```python
from build123d import *

# Parameters (mm, degrees)
SKETCH2_W                     = 520
SKETCH2_H                     = 70
BASE_FLANGE1_DEPTH            = 1
EDGE_FLANGE4_STRIP_W          = 5.4732
EDGE_FLANGE4_STRIP_H          = 1
EDGE_FLANGE4_STRIP_CUT_DEPTH  = 520
EDGE_FLANGE4_DEPTH            = 520
EDGE_FLANGE5_STRIP_W          = 5.4732
EDGE_FLANGE5_STRIP_H          = 1
EDGE_FLANGE5_STRIP_CUT_DEPTH  = 520
EDGE_FLANGE5_DEPTH            = 520
EDGE_FLANGE6_STRIP_W          = 5.4732
EDGE_FLANGE6_STRIP_H          = 1
EDGE_FLANGE6_STRIP_CUT_DEPTH  = 520
EDGE_FLANGE6_DEPTH            = 520
EDGE_FLANGE7_STRIP_W          = 5.4732
EDGE_FLANGE7_STRIP_H          = 1
EDGE_FLANGE7_STRIP_CUT_DEPTH  = 520
EDGE_FLANGE7_DEPTH            = 520
EDGE_FLANGE8_STRIP_W          = 5.4732
EDGE_FLANGE8_STRIP_H          = 1
EDGE_FLANGE8_STRIP_CUT_DEPTH  = 520
EDGE_FLANGE8_DEPTH            = 520
EDGE_FLANGE9_STRIP_W          = 5.4732
EDGE_FLANGE9_STRIP_H          = 1
EDGE_FLANGE9_STRIP_CUT_DEPTH  = 520
EDGE_FLANGE9_DEPTH            = 520
CUT_EXTRUDE2_REACH            = 527.071
CUT_EXTRUDE3_REACH            = 527.071
SKETCH38_R                    = 1.6
EDGE_FLANGE10_STRIP_W         = 5.4732
EDGE_FLANGE10_STRIP_H         = 1
EDGE_FLANGE10_STRIP_CUT_DEPTH = 520
EDGE_FLANGE10_DEPTH           = 520
HOLE1_START                   = 47
HOLE1_OUTLINE_R               = 1.5
HOLE1_DEPTH                   = 1
HOLE2_START                   = 47
HOLE2_OUTLINE_R               = 1.5
HOLE2_DEPTH                   = 1
HOLE3_START                   = -70
HOLE3_OUTLINE_R               = 1.5
HOLE3_DEPTH                   = 1
HOLE4_START                   = -70
HOLE4_OUTLINE_R               = 1.5
HOLE4_DEPTH                   = 1
SKETCH47_R                    = 1.5
CUT_EXTRUDE4_DEPTH            = 3


# Read off the part's stored shape, not the designer's step: Hole1, Hole2, Hole3, Hole4
# Sheet-metal steps are written as plain solids
with BuildPart() as part:
    # Sketch2 → Base-Flange1 (new body)
    with BuildSketch(Plane(origin=(0, 0, 0), x_dir=(1, 0, 0), z_dir=(0, 1, 0))):
        with Locations((260, 35)):
            Rectangle(SKETCH2_W, SKETCH2_H)
    extrude(amount=-BASE_FLANGE1_DEPTH)

    # Edge-Flange4 strip (across the edge) → Edge-Flange4 strip cut (cut)
    with BuildSketch(Plane(origin=(0, 0, 0), x_dir=(0, 0, -1), z_dir=(1, 0, 0))):
        with Locations((-1, -0.5)):
            Rectangle(EDGE_FLANGE4_STRIP_W, EDGE_FLANGE4_STRIP_H)
    extrude(amount=EDGE_FLANGE4_STRIP_CUT_DEPTH, mode=Mode.SUBTRACT)

    # Edge-Flange4 section (across the edge) → Edge-Flange4 (add)
    with BuildSketch(Plane(origin=(0, 0, 0), x_dir=(0, 0, -1), z_dir=(1, 0, 0))):
        with BuildLine():
            Line((0, 0.7366), (0, 14))
            Line((0, 14), (1, 14))
            Line((1, 14), (1, 0.7366))
            ThreePointArc((1, 0.7366), (1.215745145, 0.215745145), (1.7366, 0))
            Line((1.7366, 0), (1.7366, -1))
            ThreePointArc((1.7366, -1), (0.508638364, -0.491361636), (0, 0.7366))
        make_face()
    extrude(amount=EDGE_FLANGE4_DEPTH)

    # Edge-Flange5 strip (across the edge) → Edge-Flange5 strip cut (cut)
    with BuildSketch(Plane(origin=(520, 14, 0), x_dir=(0, -1, 0), z_dir=(-1, 0, 0))):
        with Locations((-1, -0.5)):
            Rectangle(EDGE_FLANGE5_STRIP_W, EDGE_FLANGE5_STRIP_H)
    extrude(amount=EDGE_FLANGE5_STRIP_CUT_DEPTH, mode=Mode.SUBTRACT)

    # Edge-Flange5 section (across the edge) → Edge-Flange5 (add)
    with BuildSketch(Plane(origin=(520, 14, 0), x_dir=(0, -1, 0), z_dir=(-1, 0, 0))):
        with BuildLine():
            Line((0, 0.7366), (0, 29))
            Line((0, 29), (1, 29))
            Line((1, 29), (1, 0.7366))
            ThreePointArc((1, 0.7366), (1.215745145, 0.215745145), (1.7366, 0))
            Line((1.7366, 0), (1.7366, -1))
            ThreePointArc((1.7366, -1), (0.508638364, -0.491361636), (0, 0.7366))
        make_face()
    extrude(amount=EDGE_FLANGE5_DEPTH)

    # Edge-Flange6 strip (across the edge) → Edge-Flange6 strip cut (cut)
    with BuildSketch(Plane(origin=(520, 13, 29), x_dir=(0, 0, -1), z_dir=(-1, 0, 0))):
        with Locations((-1, -0.5)):
            Rectangle(EDGE_FLANGE6_STRIP_W, EDGE_FLANGE6_STRIP_H)
    extrude(amount=EDGE_FLANGE6_STRIP_CUT_DEPTH, mode=Mode.SUBTRACT)

    # Edge-Flange6 section (across the edge) → Edge-Flange6 (add)
    with BuildSketch(Plane(origin=(520, 13, 29), x_dir=(0, 0, -1), z_dir=(-1, 0, 0))):
        with BuildLine():
            Line((0, 0.7366), (0, 14))
            Line((0, 14), (1, 14))
            Line((1, 14), (1, 0.7366))
            ThreePointArc((1, 0.7366), (1.215745145, 0.215745145), (1.7366, 0))
            Line((1.7366, 0), (1.7366, -1))
            ThreePointArc((1.7366, -1), (0.508638364, -0.491361636), (0, 0.7366))
        make_face()
    extrude(amount=EDGE_FLANGE6_DEPTH)

    # Edge-Flange7 strip (across the edge) → Edge-Flange7 strip cut (cut)
    with BuildSketch(Plane(origin=(0, -1, 29), x_dir=(0, 1, 0), z_dir=(1, 0, 0))):
        with Locations((-1, -0.5)):
            Rectangle(EDGE_FLANGE7_STRIP_W, EDGE_FLANGE7_STRIP_H)
    extrude(amount=EDGE_FLANGE7_STRIP_CUT_DEPTH, mode=Mode.SUBTRACT)

    # Edge-Flange7 section (across the edge) → Edge-Flange7 (add)
    with BuildSketch(Plane(origin=(0, -1, 29), x_dir=(0, 1, 0), z_dir=(1, 0, 0))):
        with BuildLine():
            Line((0, 0.7366), (0, 19))
            Line((0, 19), (1, 19))
            Line((1, 19), (1, 0.7366))
            ThreePointArc((1, 0.7366), (1.215745145, 0.215745145), (1.7366, 0))
            Line((1.7366, 0), (1.7366, -1))
            ThreePointArc((1.7366, -1), (0.508638364, -0.491361636), (0, 0.7366))
        make_face()
    extrude(amount=EDGE_FLANGE7_DEPTH)

    # Edge-Flange8 strip (across the edge) → Edge-Flange8 strip cut (cut)
    with BuildSketch(Plane(origin=(0, 0, 48), x_dir=(0, 0, -1), z_dir=(1, 0, 0))):
        with Locations((-1, -0.5)):
            Rectangle(EDGE_FLANGE8_STRIP_W, EDGE_FLANGE8_STRIP_H)
    extrude(amount=EDGE_FLANGE8_STRIP_CUT_DEPTH, mode=Mode.SUBTRACT)

    # Edge-Flange8 section (across the edge) → Edge-Flange8 (add)
    with BuildSketch(Plane(origin=(0, 0, 48), x_dir=(0, 0, -1), z_dir=(1, 0, 0))):
        with BuildLine():
            Line((0, 0.7366), (0, 19))
            Line((0, 19), (1, 19))
            Line((1, 19), (1, 0.7366))
            ThreePointArc((1, 0.7366), (1.215745145, 0.215745145), (1.7366, 0))
            Line((1.7366, 0), (1.7366, -1))
            ThreePointArc((1.7366, -1), (0.508638364, -0.491361636), (0, 0.7366))
        make_face()
    extrude(amount=EDGE_FLANGE8_DEPTH)

    # Edge-Flange9 strip (across the edge) → Edge-Flange9 strip cut (cut)
    with BuildSketch(Plane(origin=(0, 19, 47), x_dir=(0, -1, 0), z_dir=(1, 0, 0))):
        with Locations((-1, -0.5)):
            Rectangle(EDGE_FLANGE9_STRIP_W, EDGE_FLANGE9_STRIP_H)
    extrude(amount=EDGE_FLANGE9_STRIP_CUT_DEPTH, mode=Mode.SUBTRACT)

    # Edge-Flange9 section (across the edge) → Edge-Flange9 (add)
    with BuildSketch(Plane(origin=(0, 19, 47), x_dir=(0, -1, 0), z_dir=(1, 0, 0))):
        with BuildLine():
            Line((0, 0.7366), (0, 14))
            Line((0, 14), (1, 14))
            Line((1, 14), (1, 0.7366))
            ThreePointArc((1, 0.7366), (1.215745145, 0.215745145), (1.7366, 0))
            Line((1.7366, 0), (1.7366, -1))
            ThreePointArc((1.7366, -1), (0.508638364, -0.491361636), (0, 0.7366))
        make_face()
    extrude(amount=EDGE_FLANGE9_DEPTH)

    # Sketch37 → Cut-Extrude2 (cut, up to next)
    with BuildSketch(Plane(origin=(0, -1, 0), x_dir=(-1, 0, 0), z_dir=(0, -1, 0)), mode=Mode.PRIVATE) as cut_extrude2_sk1:
        Polygon((-497, 14), (-23, 14), (-20, 17), (-20, 21), (-23, 24), (-497, 24), (-500, 21), (-500, 17), align=None)
    cut_extrude2_tool1 = extrude(cut_extrude2_sk1.sketch, amount=-CUT_EXTRUDE2_REACH, mode=Mode.PRIVATE) & part.part
    add(cut_extrude2_tool1.solids().sort_by_distance((260, -1, -19))[0], mode=Mode.SUBTRACT)

    # Sketch38 → Cut-Extrude3 (cut, up to next)
    with BuildSketch(Plane.XZ.offset(1), mode=Mode.PRIVATE) as cut_extrude3_sk1:
        with Locations(Location((60, -40, 0), (0, 0, 270))):
            Circle(SKETCH38_R)
    cut_extrude3_tool1 = extrude(cut_extrude3_sk1.sketch, amount=-CUT_EXTRUDE3_REACH, mode=Mode.PRIVATE) & part.part
    # Sketch38 → Cut-Extrude3 (cut, up to next)
    with BuildSketch(Plane.XZ.offset(1), mode=Mode.PRIVATE) as cut_extrude3_sk2:
        with Locations(Location((160, -40, 0), (0, 0, 270))):
            Circle(SKETCH38_R)
    cut_extrude3_tool2 = extrude(cut_extrude3_sk2.sketch, amount=-CUT_EXTRUDE3_REACH, mode=Mode.PRIVATE) & part.part
    # Sketch38 → Cut-Extrude3 (cut, up to next)
    with BuildSketch(Plane.XZ.offset(1), mode=Mode.PRIVATE) as cut_extrude3_sk3:
        with Locations(Location((260, -40, 0), (0, 0, 270))):
            Circle(SKETCH38_R)
    cut_extrude3_tool3 = extrude(cut_extrude3_sk3.sketch, amount=-CUT_EXTRUDE3_REACH, mode=Mode.PRIVATE) & part.part
    # Sketch38 → Cut-Extrude3 (cut, up to next)
    with BuildSketch(Plane.XZ.offset(1), mode=Mode.PRIVATE) as cut_extrude3_sk4:
        with Locations(Location((360, -40, 0), (0, 0, 270))):
            Circle(SKETCH38_R)
    cut_extrude3_tool4 = extrude(cut_extrude3_sk4.sketch, amount=-CUT_EXTRUDE3_REACH, mode=Mode.PRIVATE) & part.part
    # Sketch38 → Cut-Extrude3 (cut, up to next)
    with BuildSketch(Plane.XZ.offset(1), mode=Mode.PRIVATE) as cut_extrude3_sk5:
        with Locations(Location((460, -40, 0), (0, 0, 270))):
            Circle(SKETCH38_R)
    cut_extrude3_tool5 = extrude(cut_extrude3_sk5.sketch, amount=-CUT_EXTRUDE3_REACH, mode=Mode.PRIVATE) & part.part
    add(cut_extrude3_tool1.solids().sort_by_distance((60, -1, -40))[0], mode=Mode.SUBTRACT)
    add(cut_extrude3_tool2.solids().sort_by_distance((160, -1, -40))[0], mode=Mode.SUBTRACT)
    add(cut_extrude3_tool3.solids().sort_by_distance((260, -1, -40))[0], mode=Mode.SUBTRACT)
    add(cut_extrude3_tool4.solids().sort_by_distance((360, -1, -40))[0], mode=Mode.SUBTRACT)
    add(cut_extrude3_tool5.solids().sort_by_distance((460, -1, -40))[0], mode=Mode.SUBTRACT)

    # Edge-Flange10 strip (across the edge) → Edge-Flange10 strip cut (cut)
    with BuildSketch(Plane(origin=(520, 0, -70), x_dir=(0, 0, 1), z_dir=(-1, 0, 0))):
        with Locations((-1, -0.5)):
            Rectangle(EDGE_FLANGE10_STRIP_W, EDGE_FLANGE10_STRIP_H)
    extrude(amount=EDGE_FLANGE10_STRIP_CUT_DEPTH, mode=Mode.SUBTRACT)

    # Edge-Flange10 section (across the edge) → Edge-Flange10 (add)
    with BuildSketch(Plane(origin=(520, 0, -70), x_dir=(0, 0, 1), z_dir=(-1, 0, 0))):
        with BuildLine():
            Line((0, 0.7366), (0, 18.7366))
            Line((0, 18.7366), (1, 18.7366))
            Line((1, 18.7366), (1, 0.7366))
            ThreePointArc((1, 0.7366), (1.215745145, 0.215745145), (1.7366, 0))
            Line((1.7366, 0), (1.7366, -1))
            ThreePointArc((1.7366, -1), (0.508638364, -0.491361636), (0, 0.7366))
        make_face()
    extrude(amount=EDGE_FLANGE10_DEPTH)

    # Hole1 outline → Hole1 (cut)
    with BuildSketch(Plane.XY.offset(HOLE1_START)):
        with Locations((8, 7)):
            Circle(HOLE1_OUTLINE_R)
    extrude(amount=HOLE1_DEPTH, mode=Mode.SUBTRACT)

    # Hole2 outline → Hole2 (cut)
    with BuildSketch(Plane.XY.offset(HOLE2_START)):
        with Locations((512, 7)):
            Circle(HOLE2_OUTLINE_R)
    extrude(amount=HOLE2_DEPTH, mode=Mode.SUBTRACT)

    # Hole3 outline → Hole3 (cut)
    with BuildSketch(Plane.XY.offset(HOLE3_START)):
        with Locations((512, 7)):
            Circle(HOLE3_OUTLINE_R)
    extrude(amount=HOLE3_DEPTH, mode=Mode.SUBTRACT)

    # Hole4 outline → Hole4 (cut)
    with BuildSketch(Plane.XY.offset(HOLE4_START)):
        with Locations((8, 7)):
            Circle(HOLE4_OUTLINE_R)
    extrude(amount=HOLE4_DEPTH, mode=Mode.SUBTRACT)

    # Sketch47 → Cut-Extrude4 (cut)
    with BuildSketch(Plane(origin=(0, 13, 0), x_dir=(-1, 0, 0), z_dir=(0, -1, 0))):
        with Locations(Location((-500, -13.2634, 0), (0, 0, 90))):
            Circle(SKETCH47_R)
        with Locations(Location((-440, -13.2634, 0), (0, 0, 90))):
            Circle(SKETCH47_R)
        with Locations(Location((-380, -13.2634, 0), (0, 0, 90))):
            Circle(SKETCH47_R)
        with Locations(Location((-320, -13.2634, 0), (0, 0, 90))):
            Circle(SKETCH47_R)
        with Locations(Location((-260, -13.2634, 0), (0, 0, 90))):
            Circle(SKETCH47_R)
        with Locations(Location((-200, -13.2634, 0), (0, 0, 90))):
            Circle(SKETCH47_R)
        with Locations(Location((-140, -13.2634, 0), (0, 0, 90))):
            Circle(SKETCH47_R)
        with Locations(Location((-80, -13.2634, 0), (0, 0, 90))):
            Circle(SKETCH47_R)
        with Locations(Location((-20, -13.2634, 0), (0, 0, 90))):
            Circle(SKETCH47_R)
    extrude(amount=-CUT_EXTRUDE4_DEPTH, mode=Mode.SUBTRACT)


solid = part.part
```
Here's how the part is built. I have some questions about the finished solid (model axes, mm). A direction names the side the tool comes from. Round coordinates to 2 decimals unless told otherwise and drop trailing zeros. Loops run counter-clockwise (first coordinate to the right, second up) from the corner with the lowest first, then second, coordinate; pieces in that order, holes last.
1. Thinking about a two-plate mould opening in Z: for faces 6 (the face through (264, 7, 29)), 7 (the face through (264, 10, -70)), 8 (the face through (0, 13.5, 6.8)), which applies, released by +Z, released by -Z, zero draft, split by the parting line, or undercut?
Answers:
face 6: undercut
face 7: released by -Z
face 8: zero draft
2. Will these pins go through, and if not, where does the flat tip stop? pin 1 (5 mm diameter, centred on x = 360, z = -40, fed in from -Y); pin 2 (6 mm diameter, centred on y = 5, z = -51.5, fed in from +X); pin 3 (3.5 mm diameter, centred on x = 140, z = 13.26, fed in from +Y); pin 4 (3.5 mm diameter, centred on x = 80, z = 13.26, fed in from -Y).
Answers:
pin 1: stops at y = -1
pin 2: passes through
pin 3: stops at y = 14
pin 4: stops at y = 13
3. If I drill on probe 1 along X at (y, z) = (-0.15, -40); probe 2 along Z at (x, y) = (358.5, 6.5); probe 3 along Y at (x, z) = (85.5, 37.5), over which ranges is the centre line in solid material (lowest first)?
Answers:
probe 1: x = 0 to 58.4, 61.6 to 158.4, 161.6 to 258.4, 261.6 to 358.4, 361.6 to 458.4, 461.6 to 520
probe 2: z = -70 to -69, -1 to 0, 28 to 29, 47 to 48
probe 3: y = -1 to 0, 18 to 19
4. For faces 1 (the face through (264, 6, 28)), 2 (the face through (256, 18, 40)), 3 (the face through (256, 0, -35)), 4 (the face through (256, 9, 48)), 5 (the face through (256, 19, 40)), which set-ups out of +Z, -Z, +X, -X, +Y, -Y let a thin tool reach every point of the face, with its end or its side?
Answers:
face 1: +X, -X, -Y
face 2: +X, -X
face 3: +X, -X, +Y
face 4: +Z, +X, -X, +Y, -Y
face 5: +Z, -Z, +X, -X, +Y
5. Suppose I cut it at A-A, the plane z = -50. Please give me the cut outline in (x, y).
Answers:
outline: (0, -1) - (520, -1) - (520, 0) - (0, 0) - close
